Autodesk Inventor part; units mm, degrees
ref_plane "YZ Plane" through (0, 0, 0) normal (1, 0, 0) x (0, 1, 0)
ref_plane "XZ Plane" through (0, 0, 0) normal (0, 1, 0) x (-1, 0, 0)
ref_plane "XY Plane" through (0, 0, 0) normal (0, 0, 1) x (1, 0, 0)
sketch "Sketch1" plane through (0, 0, 0) normal (0, 1, 0) x (-1, 0, 0)
  line L0 (-4.5, 24) -> (4.5, 24)
  line L1 (4.5, 24) -> (4.5, -24)
  line L2 (4.5, -24) -> (-4.5, -24)
  line L3 (-4.5, -24) -> (-4.5, 24)
  line L4 (-4.5, 24) -> (4.5, -24) construction
  line L5 (4.5, 24) -> (-4.5, -24) construction
  point P0 (0, 0)
  dimension "d0" = 9
  dimension "d1" = 48
extrude "Extrusion1" add sketch "Sketch1" along normal blind 4
sketch "Sketch2" plane through (0, 4, 0) normal (0, 1, 0) x (1, 0, 0)
  line L0 (4.5, 24) -> (-4.5, 24)
  line L1 (-4.5, 24) -> (-0.5, 24)
  line L2 (-0.5, 24) -> (-0.5, 18)
  line L3 (-0.5, 18) -> (-4.5, 18)
  line L4 (-4.5, 18) -> (-4.5, 24)
  line L5 (-4.5, -24) -> (4.5, -24)
  line L6 (-4.5, -24) -> (-0.5, -24)
  line L7 (-0.5, -24) -> (-0.5, -18)
  line L8 (-0.5, -18) -> (-4.5, -18)
  line L9 (-4.5, -18) -> (-4.5, -24)
  point P0 (0, 0)
  dimension "d4" = 4
  dimension "d5" = 6
  dimension "d6" = 4
  dimension "d7" = 6
extrude "Extrusion2" add sketch "Sketch2" along normal blind 24.5
sketch "Sketch3" plane through (0, 4, 0) normal (0, 1, 0) x (1, 0, 0)
  point P0 (0, 0)
sketch "Sketch4" plane through (0, 4, 0) normal (0, 1, 0) x (1, 0, 0)
  line L0 (-4.5, 18) -> (1, 18)
  line L1 (1, 18) -> (1, -18)
  line L2 (1, -18) -> (-4.5, -18)
  line L3 (-4.5, -18) -> (-4.5, 18)
  line L4 (-4.5, 18) -> (-4.5, -18)
  line L5 (-4.5, -18) -> (-0.5, -18)
  point P0 (0, 0)
  dimension "d10" = 5.5
  dimension "d11" = 36
extrude "Extrusion3" cut sketch "Sketch4" against normal blind 4
sketch "Sketch5" plane through (1, 4, -18) normal (-1, 0, 0) x (0, 0, 1)
  line L0 (36, -4) -> (0, -4)
  line L1 (0, -4) -> (0, 0)
  line L2 (0, 0) -> (36, 0)
  line L3 (36, 0) -> (36, -4)
  line L4 (0, 0) -> (36, 0)
  line L5 (0, 0) -> (0, -4)
  point P0 (18, -4)
  dimension "d14" = 36
  dimension "d15" = 4
extrude "Extrusion4" add sketch "Sketch5" along normal blind 2
sketch "Sketch6" plane through (0, 28.5, 0) normal (0, 1, 0) x (1, 0, 0)
  point P0 (0, 0)
sketch "Sketch7" plane through (0, 28.5, 0) normal (0, 1, 0) x (1, 0, 0)
  line L0 (-4.5, -18) -> (-4.5, -24)
  line L1 (-0.5, -18) -> (-0.5, -24)
  line L2 (-4.5, -24) -> (-0.5, -24)
  line L3 (-0.5, -24) -> (-0.5, -18)
  line L4 (-0.5, -18) -> (-4.5, -18)
  line L5 (-4.5, -18) -> (-4.5, -24)
  line L6 (-4.5, 24) -> (-4.5, 18)
  line L7 (-0.5, 24) -> (-0.5, 18)
  line L8 (-4.5, 18) -> (-0.5, 18)
  line L9 (-0.5, 18) -> (-0.5, 24)
  line L10 (-0.5, 24) -> (-4.5, 24)
  line L11 (-4.5, 24) -> (-4.5, 18)
  point P0 (0, 0)
extrude "Extrusion5" add sketch "Sketch7" along normal blind 4
properties part number "roof4"
The listing builds one solid part. Answer for the finished solid, in the listing's coordinates (mm). A direction names the side the tool comes from. Coordinates: 2 decimals unless noted, no trailing zeros. Write each loop counter-clockwise with the first axis right and the second up, starting at its lowest first coordinate (ties: lowest second). Pieces come first, ordered by that corner, then holes. Notation, with made-up numbers: (56.5, 25.25) - (61.5, 25.25) arc R21 ccw to (61.5, 45.25) - close; hole circle Ø6 at (89.5, 20.5). An arc over 180 degrees is marked (long way). One line per item, written item: value.
1) Consider line 1 along Z through (x, y) = (-1, 17); line 2 along Y through (x, z) = (1, -15.5); line 3 along X through (y, z) = (2, -7.5). Determine where each line is inside the solid, lowest interval first. Write a range as from..to.
Geometry check:
line 1: z = -24..-18, 18..24
line 2: y = 0..4
line 3: x = -1..4.5
2) For a pull along Z with two mould halves and no side action, classify faces 4 (the flat face through (-2, 16, 24)), 5 (the flat face through (4.5, 2, 0)), 6 (the flat face through (-3, 16, -18)) as pulls with the +Z half, pulls with the -Z half, needs draft (parallel to the pull), parting line crosses it, or undercut.
Geometry check:
face 4: pulls with the +Z half
face 5: needs draft
face 6: undercut
3) Find section A-A (y = 15.5). Give the vertices of the cut face in (x, z), and give its area (3 significant figures).
Geometry check:
outline: (-4.5, -24) - (-0.5, -24) - (-0.5, -18) - (-4.5, -18) - close; (-4.5, 18) - (-0.5, 18) - (-0.5, 24) - (-4.5, 24) - close
area: 48.0 mm2
4) Find section B-B (x = -2). Give the vertices of the cut face in (y, z).
Geometry check:
outline: (0, -24) - (32.5, -24) - (32.5, -18) - (0, -18) - close; (0, 18) - (32.5, 18) - (32.5, 24) - (0, 24) - close
5) Each of these flat-tipped pins is pushed along its axis until it touches: pin 1 Ø3 at (x, z) = (-1.5, 7) entering from -Y; pin 2 Ø2 at (y, z) = (2, 2) entering from -X; pin 3 Ø5 at (y, z) = (16, 20.5) entering from +X; pin 4 Ø1.6 at (x, z) = (0.5, 5.5) entering from +Y. Where does it stop, or does it pass through?
Geometry check:
pin 1: stops at y = 0
pin 2: stops at x = -1
pin 3: stops at x = -0.5
pin 4: stops at y = 4
6) A tool of negligible diameter and unlimited length cuts with its end or side. For faces 1 (the flat face through (1, 0, 0)), 2 (the flat face through (-0.5, 18, 21)), 3 (the flat face through (-1, 2, 0)), from which of +Z, -Z, +X, -X, +Y, -Y can it reach the whole face along a straight path? Write none if from no direction.
Geometry check:
face 1: +Z, -Z, +X, -X, -Y
face 2: +Z, -Z, +X, +Y
face 3: -X, +Y, -Y
7) Find section D-D (x = 0.25). Give the vertices of the cut face in (y, z), and give its area (3 significant figures).
Geometry check:
outline: (0, -24) - (4, -24) - (4, 24) - (0, 24) - close
area: 192 mm2
8) Find section C-C (y = 3.5). Give the vertices of the cut face in (x, z).
Geometry check:
outline: (-4.5, -24) - (4.5, -24) - (4.5, 24) - (-4.5, 24) - (-4.5, 18) - (-1, 18) - (-1, -18) - (-4.5, -18) - close
